Can you work these out from the model? Positions are in its coordinate system, mm. A direction names the side the tool comes from. Coordinates: 2 decimals unless noted, no trailing zeros. Order: outer loops, then holes, each group sorted by start corner. A loop starts at its lowest first (then second) coordinate and runs counter-clockwise, first axis right, second up. Notation, with made-up numbers: M -29,62.25 L 2,62.25 A20 ccw 2,100.25 Z; hole C 21,-1 d11. An arc over 180 degrees is marked long. Answer as a JSON object with one key per item and string values.
from build123d import *

# Parameters (mm, degrees)
SKETCH1_W                      = 150
SKETCH1_H                      = 180
BOSS_EXTRUDE1_DEPTH            = 12
F_3_0MM_DOWEL_HOLE1_AT_2_COUNT = 2
F_3_0MM_DOWEL_HOLE1_AT_2_PITCH = 50
F_3_0MM_DOWEL_HOLE1_AT_3_COUNT = 2
F_3_0MM_DOWEL_HOLE1_AT_3_PITCH = 100
F_3_0MM_DOWEL_HOLE1_AT_4_COUNT = 2
F_3_0MM_DOWEL_HOLE1_AT_4_PITCH = 50
BOSS_EXTRUDE2_DEPTH            = 12
FILLET4_R                      = 3
CUT_EXTRUDE1_START             = -12
SKETCH14_W                     = 60
SKETCH14_H                     = 85
CUT_EXTRUDE1_DEPTH             = 7
SKETCH17_R                     = 1.25
CUT_EXTRUDE2_DEPTH             = 132.493453829
SKETCH18_W                     = 9
SKETCH18_H                     = 185.579893617
CUT_EXTRUDE3_DEPTH             = 7.5
M3_CLEARANCE_HOLE1_D           = 3.2
M3_CLEARANCE_HOLE2_D           = 3.2


with BuildPart() as part:
    # Sketch1 → Boss-Extrude1 (new body)
    with BuildSketch(Plane(origin=(0, 0, 0), x_dir=(1, 0, 0), z_dir=(0, 1, 0))):
        Rectangle(SKETCH1_W, SKETCH1_H)
    extrude(amount=BOSS_EXTRUDE1_DEPTH)

    # Sketch6 → Ø3.0mm Dowel Hole1 (revolve, cut)
    with BuildSketch(Plane(origin=(75, 4.5, 25), x_dir=(0, 0, -1), z_dir=(0, 1, 0))):
        Polygon((0, 0), (0, 5.901290929), (1.5, 5), (1.5, 0), align=None)
    f_3_0mm_dowel_hole1 = revolve(axis=Axis((81.35, 4.5, 25), (-1, 0, 0)), mode=Mode.SUBTRACT)

    # Ø3.0mm Dowel Hole1 at 2: Ø3.0mm Dowel Hole1 ×2
    with Locations(*[(0, 0, i * F_3_0MM_DOWEL_HOLE1_AT_2_PITCH) for i in range(1, F_3_0MM_DOWEL_HOLE1_AT_2_COUNT)]):
        add(f_3_0mm_dowel_hole1, mode=Mode.SUBTRACT)

    # Ø3.0mm Dowel Hole1 at 3: Ø3.0mm Dowel Hole1 ×2
    with Locations(*[(0, 0, -i * F_3_0MM_DOWEL_HOLE1_AT_3_PITCH) for i in range(1, F_3_0MM_DOWEL_HOLE1_AT_3_COUNT)]):
        add(f_3_0mm_dowel_hole1, mode=Mode.SUBTRACT)

    # Ø3.0mm Dowel Hole1 at 4: Ø3.0mm Dowel Hole1 ×2
    with Locations(*[(0, 0, -i * F_3_0MM_DOWEL_HOLE1_AT_4_PITCH) for i in range(1, F_3_0MM_DOWEL_HOLE1_AT_4_COUNT)]):
        add(f_3_0mm_dowel_hole1, mode=Mode.SUBTRACT)

    # Mirror1: Ø3.0mm Dowel Hole1 across plane
    add(f_3_0mm_dowel_hole1.mirror(Plane(origin=(0, 0, 0), x_dir=(0, 0, 1), z_dir=(1, 0, 0))), mode=Mode.SUBTRACT)

    # Mirror1 copy 1 sketch → Mirror1 copy 1 (revolve, cut)
    with BuildSketch(Plane(origin=(-75, 4.5, 75), x_dir=(0, 0, -1), z_dir=(0, 1, 0))):
        Polygon((0, 0), (0, -5.901290929), (1.5, -5), (1.5, 0), align=None)
    revolve(axis=Axis((-81.35, 4.5, 75), (-1, 0, 0)), mode=Mode.SUBTRACT)

    # Mirror1 copy 2 sketch → Mirror1 copy 2 (revolve, cut)
    with BuildSketch(Plane(origin=(-75, 4.5, -75), x_dir=(0, 0, -1), z_dir=(0, 1, 0))):
        Polygon((0, 0), (0, -5.901290929), (1.5, -5), (1.5, 0), align=None)
    revolve(axis=Axis((-81.35, 4.5, -75), (-1, 0, 0)), mode=Mode.SUBTRACT)

    # Mirror1 copy 3 sketch → Mirror1 copy 3 (revolve, cut)
    with BuildSketch(Plane(origin=(-75, 4.5, -25), x_dir=(0, 0, -1), z_dir=(0, 1, 0))):
        Polygon((0, 0), (0, -5.901290929), (1.5, -5), (1.5, 0), align=None)
    revolve(axis=Axis((-81.35, 4.5, -25), (-1, 0, 0)), mode=Mode.SUBTRACT)

    # Sketch13 → Boss-Extrude2 (add)
    with BuildSketch(Plane(origin=(0, 12, 0), x_dir=(1, 0, 0), z_dir=(0, 1, 0))):
        Polygon((-75, 90), (75, 90), (28, 107.78), (-28, 107.78), align=None)
    extrude(amount=-BOSS_EXTRUDE2_DEPTH)

    # Fillet4
    fillet4_edges = [part.edges().sort_by_distance(p)[0] for p in [
        (28, 6, -107.78),
        (-28, 6, -107.78),
    ]]
    fillet(fillet4_edges, radius=FILLET4_R)

    # Sketch14 → Cut-Extrude1 (cut)
    with BuildSketch(Plane(origin=(0, 12, 0), x_dir=(1, 0, 0), z_dir=(0, 1, 0)).offset(CUT_EXTRUDE1_START)):
        with Locations((0, 65.28)):
            Rectangle(SKETCH14_W, SKETCH14_H)
    extrude(amount=CUT_EXTRUDE1_DEPTH, mode=Mode.SUBTRACT)

    # Sketch17 → Cut-Extrude2 (cut, through all)
    with BuildSketch(Plane(origin=(0, 7, 0), x_dir=(-1, 0, 0), z_dir=(0, -1, 0))):
        with Locations(Location((25.5, 99, 0), (0, 0, 90))):
            Circle(SKETCH17_R)
        with Locations(Location((-23.5, 99, 0), (0, 0, 90))):
            Circle(SKETCH17_R)
        with Locations(Location((25.5, 41, 0), (0, 0, 90))):
            Circle(SKETCH17_R)
        with Locations(Location((-23.5, 41, 0), (0, 0, 90))):
            Circle(SKETCH17_R)
    extrude(amount=-CUT_EXTRUDE2_DEPTH, mode=Mode.SUBTRACT)

    # Sketch18 → Cut-Extrude3 (cut)
    with BuildSketch(Plane.XZ):
        with Locations((64.75, -2.789946809)):
            Rectangle(SKETCH18_W, SKETCH18_H)
        with Locations((-64.75, -2.789946809)):
            Rectangle(SKETCH18_W, SKETCH18_H)
    extrude(amount=-CUT_EXTRUDE3_DEPTH, mode=Mode.SUBTRACT)

    # M3 Clearance Hole1 (through all)
    with Locations(Plane(origin=(0, 12, 0), x_dir=(1, 0, 0), z_dir=(0, 1, 0))):
        with Locations((-44.5, -83.45), (-44.5, -39.75)):
            m3_clearance_hole1 = Hole(M3_CLEARANCE_HOLE1_D / 2)

    # Mirror2: M3 Clearance Hole1 across plane
    add(m3_clearance_hole1.mirror(Plane(origin=(0, 0, 0), x_dir=(0, 0, 1), z_dir=(1, 0, 0))), mode=Mode.SUBTRACT)

    # M3 Clearance Hole2 (through all)
    with Locations(Plane(origin=(0, 12, 0), x_dir=(1, 0, 0), z_dir=(0, 1, 0))):
        with Locations((0, 0), (-22.5, -22.5), (22.5, 22.5), (22.5, -22.5), (-22.5, 22.5)):
            Hole(M3_CLEARANCE_HOLE2_D / 2)


solid = part.part
Item 1: If we mould it in two halves opening along X, with no side actions, what happens to faces 1 (the flat face through (-1, 0, 12)), 2 (the flat face through (-65, 7.5, -1)), 3 (the flat face through (52.08, 6.08, -98.67))? For each: pulls with the +X half, pulls with the -X half, needs draft (parallel to the pull), parting line crosses it, or undercut.
Answers follow:
{"face 1": "needs draft", "face 2": "undercut", "face 3": "pulls with the +X half"}
Item 2: Please list where these lines run through material, in increasing order: line 1 (X direction, y = 6.75, z = -43.5); line 2 (X direction, y = 7, z = 65.5); line 3 (X direction, y = 6, z = 83.45).
Answers follow:
{"line 1": "x = -75 to -69.25, -60.25 to -30, 30 to 60.25, 69.25 to 75", "line 2": "x = -75 to -69.25, -60.25 to 60.25, 69.25 to 75", "line 3": "x = -75 to -69.25, -60.25 to -46.1, -42.9 to 42.9, 46.1 to 60.25, 69.25 to 75"}
Item 3: I want a section at A-A, the plane z = -63. Write out the boundary of the cut face in (x, y), plus the area to 4 significant figures.
Answers follow:
{"outline": "M -75,0 L -69.25,0 L -69.25,7.5 L -60.25,7.5 L -60.25,0 L -30,0 L -30,7 L 30,7 L 30,0 L 60.25,0 L 60.25,7.5 L 69.25,7.5 L 69.25,0 L 75,0 L 75,12 L -75,12 Z", "area": "1,245 mm^2"}
Item 4: I want a section at C-C, the plane x = -57. Write out the boundary of the cut face in (y, z).
Answers follow:
{"outline": "M 0,-96.81 L 12,-96.81 L 12,90 L 0,90 Z"}
Item 5: I want a section at B-B, the plane z = 65. Write out the boundary of the cut face in (x, y).
Answers follow:
{"outline": "M -75,0 L -69.25,0 L -69.25,7.5 L -60.25,7.5 L -60.25,0 L 60.25,0 L 60.25,7.5 L 69.25,7.5 L 69.25,0 L 75,0 L 75,12 L -75,12 Z"}
Item 6: Which directions (+Z, -Z, +X, -X, +Y, -Y) give clear straight access to the entire face, cutting with the end or side of a thin tool? Please do faces 4 (the flat face through (69.25, 4, -2)), 5 (the flat face through (27, 3, -22.78)), 6 (the flat face through (-1, 6, 90)).
Answers follow:
{"face 4": "+Z, -Z, -Y", "face 5": "-Z, -Y", "face 6": "+Z, +X, -X, +Y, -Y"}
Item 7: I'm going to push flat-ended pins straight in: pin 1 (3 mm diameter, centred on x = -22.5, z = 22.5, fed in from -Y); pin 2 (3 mm diameter, centred on x = -25.5, z = -41, fed in from -Y); pin 3 (2.5 mm diameter, centred on y = 4.5, z = 25, fed in from +X); pin 4 (4.5 mm diameter, centred on x = 28, y = 2, fed in from -Z). Where does each tip first touch, or does it pass through?
Answers follow:
{"pin 1": "passes through", "pin 2": "stops at y = 7", "pin 3": "stops at x = 69.85", "pin 4": "stops at z = -107.02"}
